Answer from the drawing. Dimensions are ordinates in mm from the lowest x, y and z of the part. A direction names the side the tool comes from. Coordinates: 2 decimals unless noted, no trailing zeros. Write each loop counter-clockwise with the first axis right and the second up, starting at its lowest first coordinate (ties: lowest second). Pieces come first, ordered by that corner, then holes.
(1) The mould has two halves that part along Y. Classify the marked faces 3, 4 and 5: +Y half, -Y half, draft (parallel to the pull), parting line (faces both ways), or undercut.
(2) Which of the six approach directions +Z, -Z, +X, -X, +Y, -Y give full straight-line access (tool end or side, diameter ignored) to the marked faces 1 and 2?
(3) Section C-C on z = 34 is taken. Write down the section's boundary in (x, y) (1 decimal).
(4) Section B-B on y = 33 is taken. Write down the section's boundary in (x, z) (1 decimal).
(5) Section A-A on x = 10 is taken. Write down the section's boundary in (y, z) (1 decimal), then the cut area to 3 significant figures.
(6) Find the intervals of material crossed by probe 1 along X at (y, z) = (40, 40.5) (1 decimal); probe 2 along X at (y, z) = (31.5, 12) (1 decimal); probe 3 along Z at (x, y) = (76, 53), in increasing order.
(7) Section D-D on z = 7.5 is taken. Write down the section's boundary in (x, y) (1 decimal).
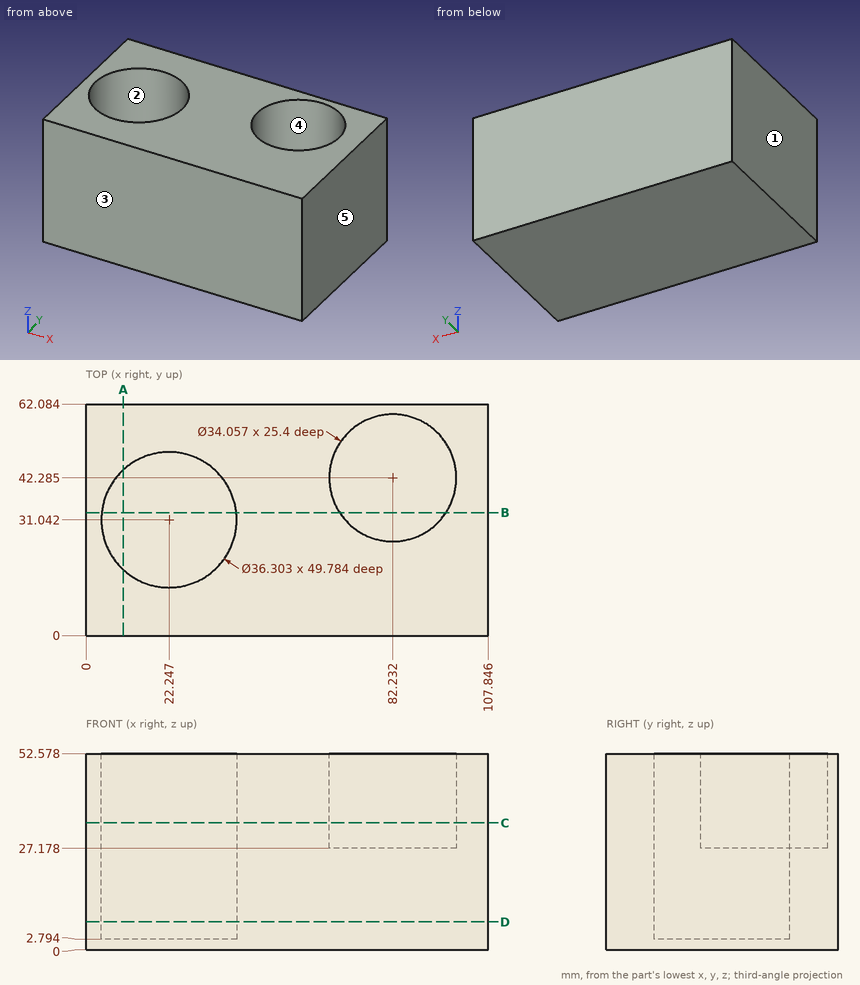
Response:
1. face 3: -Y half
1. face 4: undercut
1. face 5: draft
2. face 1: +Z, -Z, -X, +Y, -Y
2. face 2: +Z
3. outline: (0, 0) - (107.8, 0) - (107.8, 62.1) - (0, 62.1) - close; hole circle Ø36.3 at (22.2, 31); hole circle Ø34.1 at (82.2, 42.3)
4. outline: (0, 0) - (107.8, 0) - (107.8, 52.6) - (96.5, 52.6) - (96.5, 27.2) - (68, 27.2) - (68, 52.6) - (40.3, 52.6) - (40.3, 2.8) - (4.2, 2.8) - (4.2, 52.6) - (0, 52.6) - close
5. outline: (0, 0) - (62.1, 0) - (62.1, 52.6) - (44.4, 52.6) - (44.4, 2.8) - (17.6, 2.8) - (17.6, 52.6) - (0, 52.6) - close
5. area: 1,930 mm2
6. probe 1: x = 0 to 6.5, 38 to 65.4, 99.1 to 107.8
6. probe 2: x = 0 to 4.1, 40.4 to 107.8
6. probe 3: z = 0 to 27.18
7. outline: (0, 0) - (107.8, 0) - (107.8, 62.1) - (0, 62.1) - close; hole circle Ø36.3 at (22.2, 31)
